Geometry: final body of the model. Coordinates: model frame, mm. Face numbers are marked on the shaded views. A direction names the side the tool comes from. Coordinates: 2 decimals unless noted, no trailing zeros. Loops run counter-clockwise (first coordinate to the right, second up) from the corner with the lowest first, then second, coordinate; pieces in that order, holes last. Notation, with made-up numbers: (47, -3.5) - (56, -3.5) arc R19 ccw to (56, 13.5) - close; hole circle Ø3 at (43, 43). An arc over 180 degrees is marked (long way). Return JSON: item names as keys, results as strings.
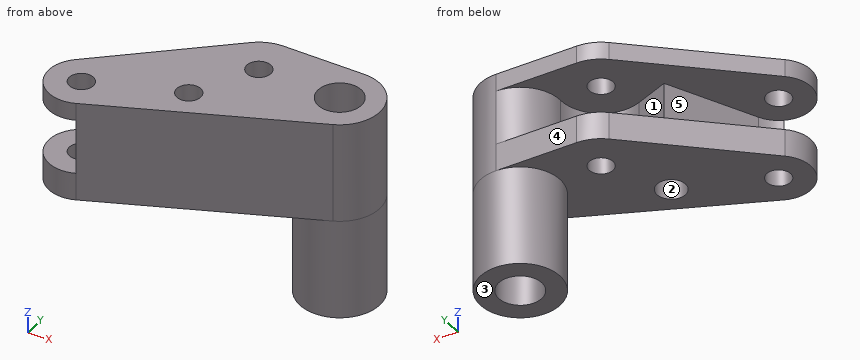
from build123d import *
from build123d.topology import SkipClean

# Parameters (mm, degrees)
SKETCH1_R           = 1.905
SKETCH1_R_2         = 3.429
BOSS_EXTRUDE1_DEPTH = 15.875
CUT_EXTRUDE2_DEPTH  = 4.365625
SKETCH6_R           = 6.35
SKETCH6_R_2         = 3.429
BOSS_EXTRUDE2_DEPTH = 15.875
SKETCH7_R           = 1.905
CUT_EXTRUDE4_DEPTH  = 45.765288281
SKETCH8_R           = 2.286
CUT_EXTRUDE5_DEPTH  = 4.365625


with BuildPart() as part:
    # Sketch1 → Boss-Extrude1 (new body)
    with BuildSketch(Plane.XY):
        with BuildLine():
            Line((-29.633029251, -19.50753994), (2.485871029, -5.843196491))
            ThreePointArc((2.485871029, -5.843196491), (6.22200923, 1.268503505), (0, 6.35))
            Line((0, 6.35), (-12.7, 6.35))
            ThreePointArc((-12.7, 6.35), (-14.910911787, 5.952677471), (-16.845147964, 4.810431203))
            Line((-16.845147964, 4.810431203), (-35.020732183, -10.851467439))
            ThreePointArc((-35.020732183, -10.851467439), (-36.033014448, -17.486271287), (-29.633029251, -19.50753994))
        make_face()
        with Locations((-12.7, 0)):
            Circle(SKETCH1_R, mode=Mode.SUBTRACT)
        with Locations((-31.652799462, -14.759942791)):
            Circle(SKETCH1_R, mode=Mode.SUBTRACT)
        Circle(SKETCH1_R_2, mode=Mode.SUBTRACT)
    extrude(amount=-BOSS_EXTRUDE1_DEPTH)

    # Sketch4 → Cut-Extrude2 (cut, symmetric)
    with SkipClean():  # the faces are left unmerged after this step: merging them gives an invalid solid
        with BuildSketch(Plane.XY.offset(-7.14375)):
            with BuildLine():
                Line((0, 6.35), (-12.7, 6.35))
                ThreePointArc((-12.7, 6.35), (-14.910911787, 5.952677471), (-16.845147964, 4.810431203))
                Line((-16.845147964, 4.810431203), (-35.020732183, -10.851467439))
                ThreePointArc((-35.020732183, -10.851467439), (-36.033014448, -17.486271287), (-29.633029251, -19.50753994))
                ThreePointArc((-29.633029251, -19.50753994), (-28.131062442, -18.530422701), (-27.053869093, -17.098529939))
                Line((-27.053869093, -17.098529939), (-20.285757113, -3.788751957))
                Line((-20.285757113, -3.788751957), (-15.073987601, -5.889540124))
                ThreePointArc((-15.073987601, -5.889540124), (-9.146995726, -5.262951703), (-6.35, 0))
                ThreePointArc((-6.35, 0), (-4.490128061, 4.490128061), (0, 6.35))
            make_face()
        extrude(amount=CUT_EXTRUDE2_DEPTH, both=True, mode=Mode.SUBTRACT)

    # Sketch6 → Boss-Extrude2 (add)
    with SkipClean():  # the faces are left unmerged after this step: merging them gives an invalid solid
        with BuildSketch(Plane(origin=(0, 0, -15.875), x_dir=(-1, 0, 0), z_dir=(0, 0, -1))):
            with Locations(Location((0, 0, 0), (0, 0, 180))):
                Circle(SKETCH6_R)
            with Locations(Location((0, 0, 0), (0, 0, 180))):
                Circle(SKETCH6_R_2, mode=Mode.SUBTRACT)
        extrude(amount=BOSS_EXTRUDE2_DEPTH)

    # Sketch7 → Cut-Extrude4 (cut, through all)
    with SkipClean():  # the faces are left unmerged after this step: merging them gives an invalid solid
        with BuildSketch(Plane(origin=(0, 0, -15.875), x_dir=(-1, 0, 0), z_dir=(0, 0, -1))):
            with Locations((17.930468191, -9.560371879)):
                Circle(SKETCH7_R)
        extrude(amount=-CUT_EXTRUDE4_DEPTH, mode=Mode.SUBTRACT)

    # Sketch8 → Cut-Extrude5 (cut)
    with SkipClean():  # the faces are left unmerged after this step: merging them gives an invalid solid
        with BuildSketch(Plane(origin=(0, 0, -15.875), x_dir=(-1, 0, 0), z_dir=(0, 0, -1))):
            with Locations((17.930468191, -9.560371879)):
                Circle(SKETCH8_R)
        extrude(amount=-CUT_EXTRUDE5_DEPTH, mode=Mode.SUBTRACT)


solid = part.part
Item 1: Section query B-B, the plane z = -23. Return loops of the section in (x, y).
Worked out:
{"outline": "circle Ø12.7 at (0, 0); hole circle Ø6.86 at (0, 0)"}
Item 2: Reachability of the marked faces 4 and 5 from +Z, -Z, +X, -X, +Y, -Y: full face, straight path, thin tool, end or side. Return the list, or none.
Worked out:
{"face 4": "+Z, -Z, +X, -X, +Y", "face 5": "-X, +Y"}
Item 3: Ray query, probe 1 along X at (y, z) = (0.25, -15.5); probe 2 along Y at (x, z) = (0, -10.5); probe 3 along Z at (x, y) = (-33, -11.25) (3 decimals). Return the intervals inside material, ascending. Write a range as from..to.
Worked out:
{"probe 1": "-22.14..-14.59, -10.81..-3.42, 3.42..6.35", "probe 2": "-6.9..-3.43, 3.43..6.35", "probe 3": "-15.875..-11.509, -2.778..0"}
Item 4: Section query A-A, the plane x = -17.5. Return loops of the section in (y, z) (3 decimals).
Worked out:
{"outline": "(-14.346, -15.875) - (-11.805, -15.875) - (-11.805, -11.509) - (-11.416, -11.509) - (-11.416, 0) - (-14.346, 0) - close; (-7.705, -11.509) - (-7.315, -11.509) - (-7.315, -15.875) - (4.246, -15.875) - (4.246, -11.509) - (-4.912, -11.509) - (-4.912, -2.778) - (4.246, -2.778) - (4.246, 0) - (-7.705, 0) - close"}
Item 5: Section query D-D, the plane y = -4.75. Return loops of the section in (x, z) (3 decimals), and give its area (3 significant figures).
Worked out:
{"outline": "(-27.94, -15.875) - (-4.214, -15.875) - (-4.214, -31.75) - (4.214, -31.75) - (4.214, 0) - (-27.94, 0) - (-27.94, -2.778) - (-20.775, -2.778) - (-20.775, -11.509) - (-27.94, -11.509) - close; hole (-17.901, -11.509) - (-8.486, -11.509) - (-8.486, -2.778) - (-17.901, -2.778) - close", "area": "499 mm^2"}
Item 6: Mould query, pull axis Z, two halves, no side actions, for the marked faces 1, 2 and 3. Classes: +Z half, -Z half, draft (parallel to the pull), parting line (faces both ways), or undercut.
Worked out:
{"face 1": "undercut", "face 2": "draft", "face 3": "-Z half"}
Item 7: First-contact query: pin 1 Ø8 at (x, y) = (-26, -6) entering from -Z (3 decimals); pin 2 Ø4.5 at (x, y) = (-17.93, -9.56) entering from -Z; pin 3 Ø6 at (x, z) = (-19, -3.5) entering from +Y. Flat tips, straight axial feed; report the tip coordinate or a pass-through.
Worked out:
{"pin 1": "z = -15.875", "pin 2": "z = -11.51", "pin 3": "y = 5.37"}
Item 8: Section query C-C, the plane y = -16. Return loops of the section in (x, z) (3 decimals), and give its area (3 significant figures).
Worked out:
{"outline": "(-36.661, -15.875) - (-33.099, -15.875) - (-33.099, -11.509) - (-36.661, -11.509) - close; (-36.661, -2.778) - (-33.099, -2.778) - (-33.099, 0) - (-36.661, 0) - close; (-30.207, -15.875) - (-21.388, -15.875) - (-21.388, 0) - (-30.207, 0) - (-30.207, -2.778) - (-26.495, -2.778) - (-26.495, -11.509) - (-30.207, -11.509) - close", "area": "133 mm^2"}
